Design review of the part built by this model. Coordinates are the model's own, in mm. Face numbers are marked on the shaded views. A direction names the side the tool comes from. Round coordinates to 2 decimals unless told otherwise and drop trailing zeros. Loops run counter-clockwise (first coordinate to the right, second up) from the corner with the lowest first, then second, coordinate; pieces in that order, holes last. Notation, with made-up numbers: (12, -34.5) -> (29, -34.5) arc R27 ccw to (29, -6.5) -> close; hole circle Ø5 at (75, -30.75). An arc over 180 degrees is marked (long way). Answer as CSV lines item,"result". Start each with the question number.
Autodesk Inventor part; units mm, degrees
ref_plane "YZ Plane" through (0, 0, 0) normal (1, 0, 0) x (0, 1, 0)
ref_plane "XZ Plane" through (0, 0, 0) normal (0, 1, 0) x (-1, 0, 0)
ref_plane "XY Plane" through (0, 0, 0) normal (0, 0, 1) x (1, 0, 0)
sketch "Szkic1" plane through (0, 0, 0) normal (0, 0, 1) x (1, 0, 0)
  line L0 (0, 0) -> (10, 0)
  line L1 (10, 12) -> (0, 12)
  arc A0 (10, 0) -> (7.5, 2) centre (7.165, -0.9812) ccw
  arc A1 (2.5, 2) -> (0, 0) centre (2.835, -0.9812) ccw
  arc A2 (7.5, 10) -> (10, 12) centre (7.165, 12.9812) ccw
  arc A3 (0, 12) -> (2.5, 10) centre (2.835, 12.9812) ccw
  arc A4 (7.5, 4) -> (7.5, 2) centre (8.8251, 3) ccw
  arc A5 (2.5, 2) -> (2.5, 4) centre (1.1749, 3) ccw
  arc A6 (7.5, 10) -> (7.5, 8) centre (8.8251, 9) ccw
  arc A7 (2.5, 8) -> (2.5, 10) centre (1.1749, 9) ccw
  arc A8 (7.5, 4) -> (7.5, 8) centre (5.2639, 6) ccw
  arc A9 (2.5, 8) -> (2.5, 4) centre (4.7361, 6) ccw
  line L2 (-1.9818, -14.25) -> (12.2979, -14.25)
  dimension "d0" = 10
  dimension "d5" = 3
  dimension "d7" = 3
  dimension "d10" = 3
  dimension "d11" = 3
  dimension "d12" = 3
  dimension "d13" = 3
revolve "Obrót1" add sketch "Szkic1" angle 180 about axis through (-1.9818, -14.25, 0) along (1, 0, 0)
sketch "Szkic2" plane through (10, 0, 0) normal (0, 0, -1) x (-1, 0, 0)
  line L0 (10, 0) -> (0, 0)
  line L1 (0, 0) -> (10, 0)
  line L2 (0, 12) -> (10, 12)
  line L3 (0, 12) -> (10, 12)
  arc A0 (7.5, 10) -> (7.5, 8) centre (8.8251, 9) ccw
  line L4 (10, 12) -> (10, -40.5)
  arc A1 (2.5, 8) -> (2.5, 10) centre (1.1749, 9) ccw
  arc A2 (2.5, 8) -> (2.5, 4) centre (4.7361, 6) ccw
  arc A3 (2.5, 8) -> (2.5, 10) centre (1.175, 9) ccw
  arc A4 (7.5, 4) -> (7.5, 8) centre (5.2639, 6) ccw
  arc A5 (7.5, 10) -> (7.5, 8) centre (8.8251, 9) ccw
  arc A6 (7.5, 4) -> (7.5, 2) centre (8.8251, 3) ccw
  arc A7 (7.5, 4) -> (7.5, 8) centre (5.2639, 6) ccw
  line L5 (8.2639, 6) -> (8.2639, -34.5)
  arc A8 (2.5, 8) -> (2.5, 4) centre (4.7361, 6) ccw
  arc A9 (2.5, 2) -> (0, 0) centre (2.835, -0.9812) ccw
  arc A10 (2.5, 2) -> (2.5, 4) centre (1.1749, 3) ccw
  line L6 (2.835, 3) -> (2.835, -31.5)
  arc A11 (7.5, 4) -> (7.5, 2) centre (8.8251, 3) ccw
  arc A12 (2.5, 2) -> (0, 0) centre (2.835, -0.9812) ccw
  arc A13 (10, 0) -> (7.5, 2) centre (7.165, -0.9812) ccw
  arc A14 (10, 0) -> (7.5, 2) centre (7.165, -0.9812) ccw
  arc A15 (7.5, 10) -> (10, 12) centre (7.165, 12.9812) ccw
  arc A16 (7.5, 10) -> (10, 12) centre (7.165, 12.9812) ccw
  arc A17 (0, 12) -> (2.5, 10) centre (2.835, 12.9812) ccw
  arc A18 (0, 12) -> (2.5, 10) centre (2.835, 12.9812) ccw
  dimension "d16" = 1.66
extrude "Wyciągnięcie proste1" add sketch "Szkic2" along normal blind 25 contours L0 L5 A13 | L0 L6 A10 A2 A1 A17 L2 A15 A0 A4 A6 A13 L5 | L0 A9 A10 L6
sketch "Szkic3" plane through (10, -28.5, 0) normal (0, 0, -1) x (-1, 0, 0)
  line L0 (10, 0) -> (0, 0)
  line L1 (0, 0) -> (10, 0)
  arc A0 (2.5, -10) -> (0, -12) centre (2.835, -12.9812) ccw
  line L2 (0, -12) -> (10, -12)
  line L3 (0, -12) -> (10, -12)
  arc A1 (10, -12) -> (7.5, -10) centre (7.165, -12.9812) ccw
  arc A2 (10, -12) -> (7.5, -10) centre (7.165, -12.9812) ccw
  arc A3 (2.5, -10) -> (2.5, -8) centre (1.1749, -9) ccw
  arc A4 (2.5, -10) -> (0, -12) centre (2.835, -12.9812) ccw
  arc A5 (0, 0) -> (2.5, -2) centre (2.835, 0.9812) ccw
  arc A6 (2.5, -4) -> (2.5, -2) centre (1.1749, -3) ccw
  arc A7 (0, 0) -> (2.5, -2) centre (2.835, 0.9812) ccw
  line L4 (7.5, 30.5) -> (7.5, -2)
  arc A8 (7.5, -2) -> (10, 0) centre (7.165, 0.9812) ccw
  arc A9 (7.5, -2) -> (10, 0) centre (7.165, 0.9812) ccw
  arc A10 (7.5, -2) -> (7.5, -4) centre (8.8251, -3) ccw
  arc A11 (7.5, -2) -> (7.5, -4) centre (8.8251, -3) ccw
  arc A12 (2.5, -4) -> (2.5, -2) centre (1.1749, -3) ccw
  arc A13 (2.5, -4) -> (2.5, -8) centre (4.7361, -6) ccw
  arc A14 (2.5, -4) -> (2.5, -8) centre (4.7361, -6) ccw
  arc A15 (7.5, -8) -> (7.5, -4) centre (5.2639, -6) ccw
  arc A16 (7.5, -8) -> (7.5, -4) centre (5.2639, -6) ccw
  line L5 (7.5, 38.5) -> (7.5, -10)
  arc A17 (7.5, -8) -> (7.5, -10) centre (8.618, -9) ccw
  arc A18 (2.5, -10) -> (2.5, -8) centre (1.382, -9) ccw
  point P0 (10, 28.5)
extrude "Wyciągnięcie proste2" add sketch "Szkic3" along normal blind 25 contours A8 L4 L0 | L4 A10 L5 A17 A1 L2 A0 A18 A13 A6 A5 L0 | A15 L5
sketch "Szkic4" plane through (0, 12, 0) normal (0, 1, 0) x (1, 0, 0)
  line L0 (0, 0) -> (10, 0)
  circle A0 centre (5, 17) radius 1.75
  dimension "d22" = 3.5
extrude "Wyciągnięcie proste3" cut sketch "Szkic4" against normal blind 250
sketch "Szkic5" plane through (0, 12, 0) normal (0, 1, 0) x (1, 0, 0)
  point P0 (0, 0)
sketch "Szkic6" plane through (10, 0, -25) normal (0, 0, -1) x (-1, 0, 0)
  line L0 (10, 12) -> (0, 12)
  line L1 (5, 12) -> (5, -40.5)
  line L2 (0, -40.5) -> (10, -40.5)
  line L3 (10, -28.5) -> (0, -28.5)
  line L4 (5, -28.5) -> (15, -28.5)
  line L5 (15, -28.5) -> (15, -40.5)
  line L6 (15, -40.5) -> (5, -40.5)
  line L7 (0, 0) -> (10, 0)
  line L8 (5, 0) -> (15, 0)
  line L9 (15, 0) -> (15, 12)
  line L10 (15, 12) -> (5, 12)
  line L11 (15, -34.5) -> (12, -34.5)
  line L12 (12, -34.5) -> (12, -30)
  line L13 (12, -34.5) -> (12, -39)
  line L14 (13.5, -30) -> (10.5, -30)
  line L15 (10.5, -30) -> (10.5, -39)
  line L16 (10.5, -39) -> (13.5, -39)
  line L17 (13.5, -39) -> (13.5, -30)
  dimension "d25" = 10
  dimension "d26" = 3
  dimension "d27" = 4.5
  dimension "d28" = 4.5
  dimension "d29" = 3
extrude "Wyciągnięcie proste4" add sketch "Szkic6" along normal blind 2 contours L3 L4 L5 L6 L2 L1
sketch "Szkic7" plane through (10, 0, -25) normal (0, 0, -1) x (-1, 0, 0)
  line L0 (0, 0) -> (10, 0)
  line L1 (5, 0) -> (5, 12)
  line L2 (10, 12) -> (0, 12)
  line L3 (5, 12) -> (15, 12)
  line L4 (15, 12) -> (15, 0)
  line L5 (15, 0) -> (5, 0)
  line L6 (15, 6) -> (12, 6)
  line L7 (12, 6) -> (12, 10.5)
  line L8 (12, 6) -> (12, 1.5)
  line L9 (13.5, 10.5) -> (10.5, 10.5)
  line L10 (10.5, 10.5) -> (10.5, 1.5)
  line L11 (10.5, 1.5) -> (13.5, 1.5)
  line L12 (13.5, 1.5) -> (13.5, 10.5)
  dimension "d32" = 10
  dimension "d33" = 3
  dimension "d34" = 4.5
  dimension "d35" = 4.5
  dimension "d36" = 3
extrude "Wyciągnięcie proste5" add sketch "Szkic7" along normal blind 2
fillet "Zaokrąglenie1" radius 2 2 edges at (5, 6, -25) (5, -34.5, -25)
properties part number "obejma2"
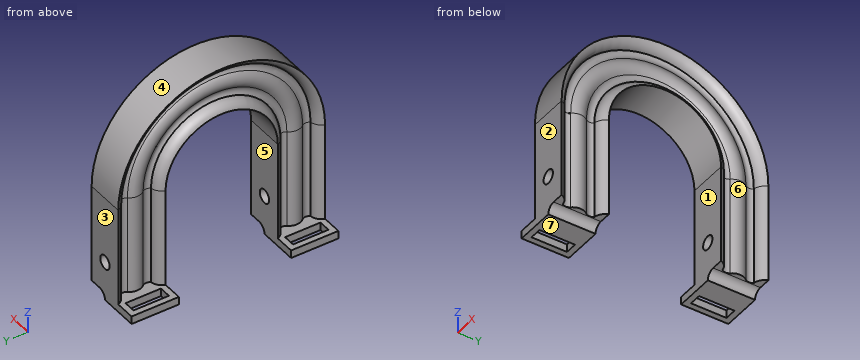
Q1. Machinability: for the marked faces 5, 6 and 7, which of the approach directions +Z, -Z, +X, -X, +Y, -Y give a long, thin tool a straight path to every point of the face, cutting with its end or side? Answer none if there is none.
Q2. Add section C-C, the plane y = -14.25. Give the boundary of the cut face in (x, z).
Q3. To check wall thickness, follow probe 1 along Y at (x, z) = (2.25, -6); probe 2 along X at (y, z) = (-32.5, -17). State the ranges of each line that lie inside material, in increasing order. Write a range as from..to.
Q4. For pin 1 Ø3 at (x, y) = (1.5, -4) entering from -Z; pin 2 Ø0.6 at (y, z) = (5, -26) entering from +X; pin 3 Ø2.5 at (x, y) = (-0.5, -33.5) entering from +Z; pin 4 Ø1.5 at (y, z) = (-1, -21.5) entering from -X, all flat-tipped, find the tip position at first contact; note any pin that passes through.
Q5. Add section A-A, the plane z = -17. State how many separate pieces and enclosed holes the cut face has, and give its area (3 significant figures).
Q6. Mouldability with a two-part tool opening along Y and no side actions: class the marked faces 1, 2, 3 and 4 as pulls with the +Y half, pulls with the -Y half, needs draft (parallel to the pull), parting line crosses it, or undercut.
Q7. Add section B-B, the plane x = -2. Give the boundary of the cut face in (y, z), and give its area (3 significant figures).
Q8. Add section D-D, the plane x = 4.25. Give the boundary of the cut face in (y, z), and give its area (3 significant figures).
Worked answers:
1,face 5,"-Z, +X, -X"
1,face 6,"-Z, +X"
1,face 7,"-Z, +X, -X, +Y, -Y"
2,outline,"(0, 14.25) -> (10, 14.25) arc R3 ccw to (7.5, 16.25) arc R1.66 cw to (7.5, 18.25) arc R3 ccw to (7.5, 22.25) arc R1.66 cw to (7.5, 24.25) arc R3 ccw to (10, 26.25) -> (0, 26.25) arc R3 ccw to (2.5, 24.25) arc R1.66 cw to (2.5, 22.25) arc R3 ccw to (2.5, 18.25) arc R1.66 cw to (2.5, 16.25) arc R3 ccw to start"
3,probe 1,"y = -40.5..-38.54, -36.18..-32.82, -30.46..-28.5, 0..1.96, 4.32..7.68, 10.04..12"
3,probe 2,"x = 2.5..3.25, 6.75..7.5"
4,pin 1,"stops at z = 8.06"
4,pin 2,"stops at x = 5.48"
4,pin 3,"stops at z = 19.01"
4,pin 4,"passes through"
5,separate pieces,"4"
5,enclosed holes,"0"
5,area,"68.6 mm^2"
6,face 1,"undercut"
6,face 2,"pulls with the -Y half"
6,face 3,"pulls with the +Y half"
6,face 4,"parting line crosses it"
7,outline,"(-40.5, -27) -> (-39, -27) -> (-39, -25) -> (-40.5, -25) -> close; (-30, -27) -> (-28.5, -27) -> (-28.5, -25) -> (-30, -25) -> close; (0, -27) -> (1.5, -27) -> (1.5, -25) -> (0, -25) -> close; (10.5, -27) -> (12, -27) -> (12, -25) -> (10.5, -25) -> close"
7,area,"12.0 mm^2"
8,outline,"(-40.5, -27) -> (-28.5, -27) -> (-28.5, -18.58) -> (-40.5, -18.58) -> close; (-40.5, -15.42) -> (-28.5, -15.42) -> (-28.5, 0) arc R14.25 cw to (0, 0) -> (0, -15.42) -> (12, -15.42) -> (12, 0) arc R26.25 ccw to (-40.5, 0) -> close; (0, -27) -> (12, -27) -> (12, -18.58) -> (0, -18.58) -> close"
8,area,"1,340 mm^2"
